Part model, mm, in its own coordinate system. Coordinates: 2 decimals unless noted, no trailing zeros. Order: outer loops, then holes, each group sorted by start corner. A loop starts at its lowest first (then second) coordinate and runs counter-clockwise, first axis right, second up. Notation, with made-up numbers: M -23,27.5 L 16,27.5 A14 ccw 16,33.5 Z; hole C 42,-24.5 d1. An arc over 180 degrees is marked long. Answer in a Markdown table with one row per item. Add a question column.
from build123d import *

# Parameters (mm, degrees)
SKETCH1_W           = 88.9
SKETCH1_H           = 76.2
SKETCH1_W_2         = 53.65
SKETCH1_H_2         = 15.65
BOSS_EXTRUDE1_DEPTH = 6.35
SKETCH2_W           = 5.334
SKETCH2_H           = 3.302
CUT_EXTRUDE1_DEPTH  = 59.887477446
SKETCH3_W           = 6.35
SKETCH3_H           = 6.35
BOSS_EXTRUDE2_DEPTH = 6.35


with BuildPart() as part:
    # Sketch1 → Boss-Extrude1 (new body)
    with BuildSketch(Plane(origin=(0, 0, 0), x_dir=(1, 0, 0), z_dir=(0, 1, 0))):
        Rectangle(SKETCH1_W, SKETCH1_H)
        with Locations((-7.465, 0)):
            Rectangle(SKETCH1_W_2, SKETCH1_H_2, mode=Mode.SUBTRACT)
    extrude(amount=BOSS_EXTRUDE1_DEPTH)

    # Sketch2 → Cut-Extrude1 (cut, through all)
    with BuildSketch(Plane(origin=(0, 0, 0), x_dir=(1, 0, 0), z_dir=(0, 1, 0))):
        with Locations((-25.4, -36.449)):
            Rectangle(SKETCH2_W, SKETCH2_H)
        with Locations((-15.24, -36.449)):
            Rectangle(SKETCH2_W, SKETCH2_H)
        with Locations((-5.08, -36.449)):
            Rectangle(SKETCH2_W, SKETCH2_H)
        with Locations((5.08, -36.449)):
            Rectangle(SKETCH2_W, SKETCH2_H)
        with Locations((15.24, -36.449)):
            Rectangle(SKETCH2_W, SKETCH2_H)
        with Locations((25.4, -36.449)):
            Rectangle(SKETCH2_W, SKETCH2_H)
        with Locations((25.4, 36.449)):
            Rectangle(SKETCH2_W, SKETCH2_H)
        with Locations((15.24, 36.449)):
            Rectangle(SKETCH2_W, SKETCH2_H)
        with Locations((5.08, 36.449)):
            Rectangle(SKETCH2_W, SKETCH2_H)
        with Locations((-5.08, 36.449)):
            Rectangle(SKETCH2_W, SKETCH2_H)
        with Locations((-15.24, 36.449)):
            Rectangle(SKETCH2_W, SKETCH2_H)
        with Locations((-25.4, 36.449)):
            Rectangle(SKETCH2_W, SKETCH2_H)
    extrude(amount=CUT_EXTRUDE1_DEPTH, mode=Mode.SUBTRACT)

    # Sketch3 → Boss-Extrude2 (add)
    with BuildSketch(Plane(origin=(0, 6.35, 0), x_dir=(1, 0, 0), z_dir=(0, 1, 0))):
        with Locations((-47.625, 34.925)):
            Rectangle(SKETCH3_W, SKETCH3_H)
        with Locations((-47.625, 22.225)):
            Rectangle(SKETCH3_W, SKETCH3_H)
        with Locations((-47.625, 9.525)):
            Rectangle(SKETCH3_W, SKETCH3_H)
        with Locations((-47.625, -9.525)):
            Rectangle(SKETCH3_W, SKETCH3_H)
        with Locations((-47.625, -22.225)):
            Rectangle(SKETCH3_W, SKETCH3_H)
        with Locations((-47.625, -34.925)):
            Rectangle(SKETCH3_W, SKETCH3_H)
        with Locations((47.625, -34.925)):
            Rectangle(SKETCH3_W, SKETCH3_H)
        with Locations((47.625, -22.225)):
            Rectangle(SKETCH3_W, SKETCH3_H)
        with Locations((47.625, -9.525)):
            Rectangle(SKETCH3_W, SKETCH3_H)
        with Locations((47.625, 9.525)):
            Rectangle(SKETCH3_W, SKETCH3_H)
        with Locations((47.625, 22.225)):
            Rectangle(SKETCH3_W, SKETCH3_H)
        with Locations((47.625, 34.925)):
            Rectangle(SKETCH3_W, SKETCH3_H)
    extrude(amount=-BOSS_EXTRUDE2_DEPTH)


solid = part.part
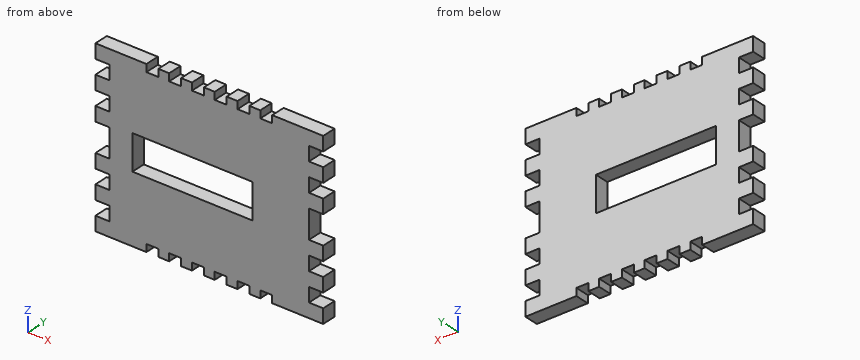
(1) Wall check: line 1 (Z direction, x = -21, y = 0.5) (3 decimals); line 2 (Z direction, x = -46, y = 4.25); line 3 (X direction, y = 2.5, z = -7.5). Give the ranges that are in metal, low to high.
(2) Slice it at C-C (z = -29.5). List the corners of the cut face in (x, y).
(3) Slice it at B-B (x = 25). List the corners of the cut face in (y, z).
(4) Slice it at A-A (x = -11.5). List the corners of the cut face in (y, z) (3 decimals).
(5) Drop flat-ended pins along their axis: P1, Ø6, axis at x = 1, z = -18.5, coming from the -Y side; P2, Ø2.5, axis at x = 26, y = 2, coming from the -Z side; P3, Ø2.5, axis at x = -26, y = 4, coming from the +Z side. Give the stop position or say it passes through.
Computed:
| question | item | result |
|---|---|---|
| 1 | line 1 | z = -38.1 to -7.825, 7.825 to 38.1 |
| 1 | line 2 | z = -38.1 to -31.75, -25.4 to -19.05, -12.7 to -6.35, 6.35 to 12.7, 19.05 to 25.4, 31.75 to 38.1 |
| 1 | line 3 | x = -50.8 to -34.29, 19.36 to 50.8 |
| 2 | outline | M -44.45,0 L 44.45,0 L 44.45,6.35 L -44.45,6.35 Z |
| 3 | outline | M 0,-34.8 L 6.35,-34.8 L 6.35,34.8 L 0,34.8 Z |
| 4 | outline | M 0,-38.1 L 6.35,-38.1 L 6.35,-7.825 L 0,-7.825 Z; M 0,7.825 L 6.35,7.825 L 6.35,38.1 L 0,38.1 Z |
| 5 | P1 | stops at y = 0 |
| 5 | P2 | stops at z = -34.8 |
| 5 | P3 | stops at z = 34.8 |
